Geometry: final body of the model. Coordinates: model frame, mm. A direction names the side the tool comes from. Coordinates: 2 decimals unless noted, no trailing zeros. Order: outer loops, then holes, each group sorted by start corner. A loop starts at its lowest first (then second) coordinate and runs counter-clockwise, first axis right, second up. Notation, with made-up numbers: M 24,10 L 36,10 A25 cw 36,48 Z; hole C -36.5,-29.75 d7. An arc over 180 degrees is marked long. One line per question, with ' | ' between items.
from build123d import *

# Parameters (mm, degrees)
F0_W     = 100
F0_H     = 100
F1_DEPTH = 15
F3_DEPTH = 5
F4_R     = 2.5
F5_DEPTH = 15.001


with BuildPart() as f1:
    # F0 (on Top) → F1 (new body)
    with BuildSketch(Plane.XY):
        Rectangle(F0_W, F0_H)
    extrude(amount=F1_DEPTH)

    # F2 (on face) → F3 (cut)
    with BuildSketch(Plane.XY.offset(15)):
        Polygon((-40, -40), (50, -40), (50, -35), (-35, -35), (-35, 35), (35, 35), (35, -15), (-15, -15), (-15, 15), (15, 15), (15, 0), (20, 0), (20, 20), (-20, 20), (-20, -20), (40, -20), (40, 40), (-40, 40), align=None)
    extrude(amount=-F3_DEPTH, mode=Mode.SUBTRACT)

    # F4 (on face) → F5 (cut, through all)
    with BuildSketch(Plane.XY.offset(15)):
        with Locations((17.5, 0)):
            Circle(F4_R)
    extrude(amount=-F5_DEPTH, mode=Mode.SUBTRACT)


solid = f1.part
1. Material intervals for line 1 (X direction, y = 0, z = 12.25); line 2 (Y direction, x = 39.5, z = 10.5); line 3 (Y direction, x = 17.5, z = 5.5), sorted ascending. Write a range as [from, to].
Response values:
line 1: x = [-50, -40], [-35, -20], [-15, 15], [20, 35], [40, 50] | line 2: y = [-50, -40], [-35, -20], [40, 50] | line 3: y = [-50, -2.5], [2.5, 50]
2. Section A-A, the plane y = 25.5. Output: boundary loops of the cut face in (x, z).
Response values:
outline: M -50,0 L 50,0 L 50,15 L 40,15 L 40,10 L 35,10 L 35,15 L -35,15 L -35,10 L -40,10 L -40,15 L -50,15 Z
3. Access query for faces 5 (the face through (-20, 0, 13)), 6 (the face through (-1, -50, 7)), 7 (the face through (8, -35, 13)). Directions: +Z, -Z, +X, -X, +Y, -Y. A direction counts if a zero-diameter tool reaches every point of the face in a straight line with its end or side. Return the directions, or none.
Response values:
face 5: +Z | face 6: +Z, -Z, +X, -X, -Y | face 7: +Z, +X
4. Pin query (flat end, axial travel): P1, Ø4, axis at x = 23.5, y = -18, coming from the -Z side; P2, Ø3, axis at x = 17.5, y = 0, coming from the -Z side. Return the tip coordinate at first contact, or that it passes through.
Response values:
P1: stops at z = 0 | P2: passes through
5. Section C-C, the plane z = 12.25. Output: boundary loops of the cut face in (x, y).
Response values:
outline: M -50,-50 L 50,-50 L 50,-40 L -40,-40 L -40,40 L 40,40 L 40,-20 L -20,-20 L -20,20 L 20,20 L 20,0 A2.5 cw 15,0 L 15,15 L -15,15 L -15,-15 L 35,-15 L 35,35 L -35,35 L -35,-35 L 50,-35 L 50,50 L -50,50 Z
6. Section D-D, the plane x = 4.5. Output: boundary loops of the cut face in (y, z).
Response values:
outline: M -50,0 L 50,0 L 50,15 L 40,15 L 40,10 L 35,10 L 35,15 L 20,15 L 20,10 L 15,10 L 15,15 L -15,15 L -15,10 L -20,10 L -20,15 L -35,15 L -35,10 L -40,10 L -40,15 L -50,15 Z
7. Section B-B, the plane x = 17.5. Output: boundary loops of the cut face in (y, z), and give its area (3 significant figures).
Response values:
outline: M -50,0 L -2.5,0 L -2.5,15 L -15,15 L -15,10 L -20,10 L -20,15 L -35,15 L -35,10 L -40,10 L -40,15 L -50,15 Z; M 2.5,0 L 50,0 L 50,15 L 40,15 L 40,10 L 35,10 L 35,15 L 20,15 L 20,10 L 2.5,10 Z | area: 1,260 mm^2
8. Draft query along Y for faces 1 (the face through (-40, 1, 13)), 2 (the face through (-1, 1, 0)), 3 (the face through (-1, 50, 7)), 4 (the face through (0, 20, 13)). Return one class per face: pulls with the +Y half, pulls with the -Y half, needs draft (parallel to the pull), parting line crosses it, or undercut.
Response values:
face 1: undercut | face 2: needs draft | face 3: pulls with the +Y half | face 4: undercut
